from build123d import *

# Parameters (mm, degrees)
F0_W        = 53
F0_H        = 33.7
F1_DEPTH    = 5.5
F2_T1_DEPTH = 68


# Not quite as in the source:
# - a fillet or chamfer that OpenCascade refuses, or shapes differently, is made with other operations: its cross-section is extruded or revolved along the edge and cut away or added


with BuildPart() as f1:
    # F0 (on Front) → F1 (new body)
    with BuildSketch(Plane.XZ):
        with Locations((-24.1282908246, 38.41047619)):
            Rectangle(F0_W, F0_H)
    extrude(amount=F1_DEPTH)

    # F2: fillet of radius 3 on 4 edges, made by hand

    # F2_s2 → F2_t1 (cut)
    with BuildSketch(Plane.YZ.offset(-58.1282908246)):
        with BuildLine():
            ThreePointArc((-2.5, 55.26047619), (-4.6213203436, 54.3817965336), (-5.5, 52.26047619))
            Line((-5.5, 52.26047619), (-5.5, 55.26047619))
            Line((-5.5, 55.26047619), (-2.5, 55.26047619))
        make_face()
        with BuildLine():
            ThreePointArc((-3, 55.26047619), (-0.8786796564, 54.3817965336), (0, 52.26047619))
            Line((0, 52.26047619), (0, 55.26047619))
            Line((0, 55.26047619), (-3, 55.26047619))
        make_face()
        with BuildLine():
            ThreePointArc((-3, 21.56047619), (-0.8786796564, 22.4391558465), (0, 24.56047619))
            Line((0, 24.56047619), (0, 21.56047619))
            Line((0, 21.56047619), (-3, 21.56047619))
        make_face()
        with BuildLine():
            ThreePointArc((-2.5, 21.56047619), (-4.6213203436, 22.4391558465), (-5.5, 24.56047619))
            Line((-5.5, 24.56047619), (-5.5, 21.56047619))
            Line((-5.5, 21.56047619), (-2.5, 21.56047619))
        make_face()
    extrude(amount=F2_T1_DEPTH, mode=Mode.SUBTRACT)


solid = f1.part
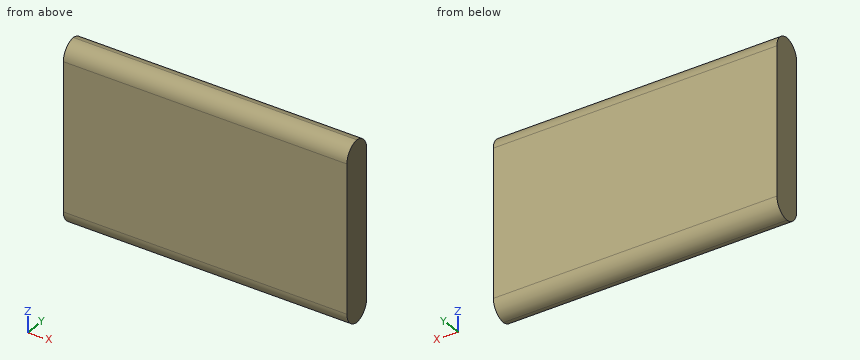
Input: part model. Units: mm. Frame: model coordinates. Coordinates: 2 decimals unless noted, no trailing zeros. Loops run counter-clockwise (first coordinate to the right, second up) from the corner with the lowest first, then second, coordinate; pieces in that order, holes last.
Q1. Cut plane C-C (z = 53). Output: boundary loops of the cut face in (x, y).
Q2. Cut plane A-A (x = -45.5). Output: boundary loops of the cut face in (y, z).
Q3. Material intervals for line 1 (Y direction, x = -36.5, z = 52.5); line 2 (Z direction, x = -42.5, y = -0.7); line 3 (Z direction, x = -26.5, y = -3.15), sorted ascending.
Q4. Cut plane B-B (y = -0.6). Output: boundary loops of the cut face in (x, z), then the cut area to 3 significant figures.
Working result:
1. outline: (-50.63, -5.41) - (2.37, -5.41) - (2.37, -0.09) - (-50.63, -0.09) - close
2. outline: (-5.5, 24.56) arc R3 ccw to (-2.75, 21.57) arc R3 ccw to (0, 24.56) - (0, 52.26) arc R3 ccw to (-2.75, 55.25) arc R3 ccw to (-5.5, 52.26) - close
3. line 1: y = -5.49 to -0.01
3. line 2: z = 22.63 to 54.19
3. line 3: z = 21.63 to 55.19
4. outline: (-50.63, 22.76) - (2.37, 22.76) - (2.37, 54.06) - (-50.63, 54.06) - close
4. area: 1,660 mm2
